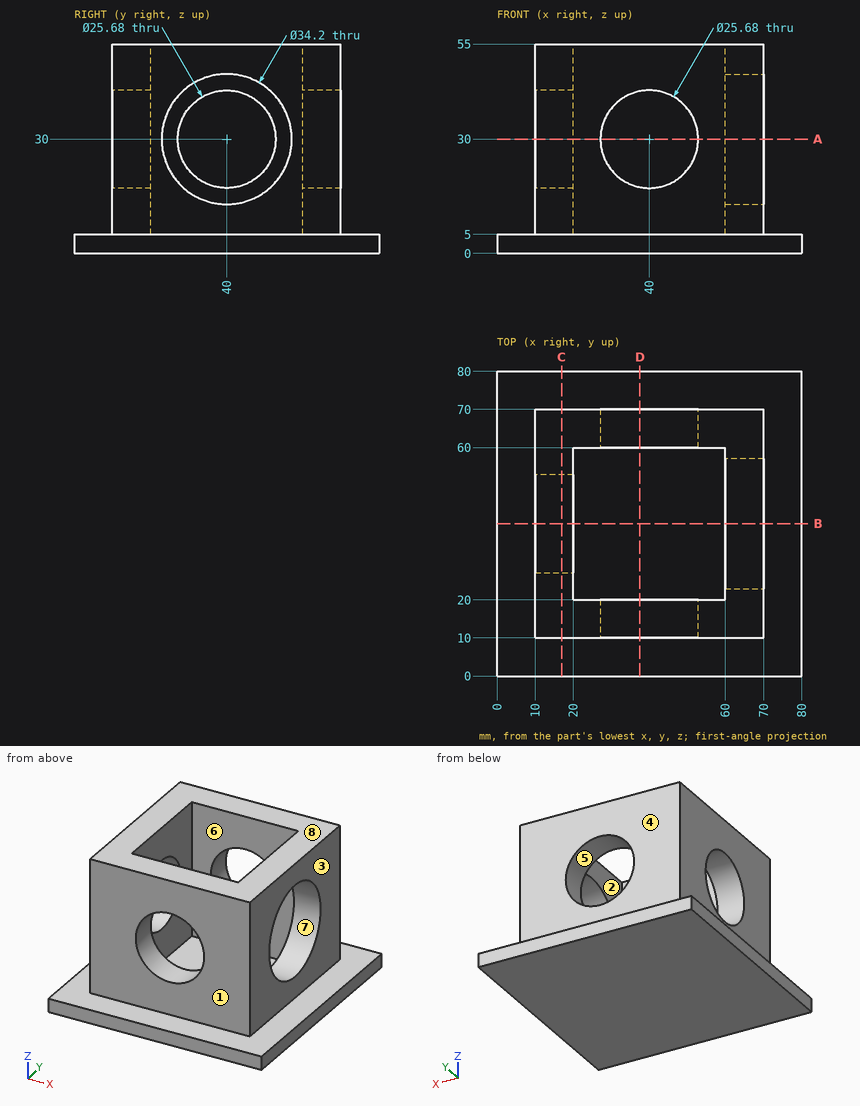
Design review of the part shown in the three views and the two pictorial views. Dimensions are in mm from the part's minimum x, y and z. A direction names the side the tool comes from. Coordinates: 2 decimals unless noted, no trailing zeros. Order: outer loops, then holes, each group sorted by start corner. A loop starts at its lowest first (then second) coordinate and runs counter-clockwise, first axis right, second up. Notation, with made-up numbers: (31.5, -11) -> (67.5, -11) arc R28 ccw to (67.5, 16) -> close; hole circle Ø5 at (57, -8.5). An arc over 180 degrees is marked (long way). Use one line per item in the form item = value. Start each with the question number.
(1) Add section D-D on x = 37.5. State the section outline as (y, z) points.
(2) The part is to be moulded in two halves that separate along Z. For the marked faces 5, 6, 7 and 8, say which applies: +Z half, -Z half, draft (parallel to the pull), parting line (faces both ways), or undercut.
(3) Add section C-C on x = 17. State the section outline as (y, z) points.
(4) For probe 1 along Y at (x, z) = (26, 40.5); probe 2 along Z at (x, y) = (63.75, 40); probe 3 along X at (y, z) = (40, 15), list the stretches that pass through material, from the lowest coordinate up.
(5) Add section B-B on y = 40. State the section outline as (x, z) points, plus the area to 3 significant figures.
(6) Insertion check: pin 1 (10 mm diameter, centred on x = 61, z = 31, fed in from -Y); pin 2 (1.5 mm diameter, centred on x = 67, y = 59.5, fed in from -Z); pin 3 (10 mm diameter, centred on y = 41, z = 48.5, fed in from +X); pin 4 (25 mm diameter, centred on x = 54.5, z = 22.5, fed in from +Y). Each pin has a flat end and moves straight along its axis. Give the tip position at first contact, or say it passes through.
(7) For the marked faces 1, 2, 3 and 4, list the 3-axis set-ups (+Z, -Z, +X, -X, +Y, -Y) from which the entire face can be reached by the end or side of a thin tool; tool diameter is ignored.
(8) Add section A-A on z = 30. State the section outline as (x, y) points, plus the area to 3 significant figures.
Answer block:
q1.outline = (0, 0) -> (80, 0) -> (80, 5) -> (70, 5) -> (70, 17.41) -> (60, 17.41) -> (60, 5) -> (20, 5) -> (20, 17.41) -> (10, 17.41) -> (10, 5) -> (0, 5) -> close; (10, 42.59) -> (20, 42.59) -> (20, 55) -> (10, 55) -> close; (60, 42.59) -> (70, 42.59) -> (70, 55) -> (60, 55) -> close
q2.face_5 = undercut
q2.face_6 = draft
q2.face_7 = undercut
q2.face_8 = +Z half
q3.outline = (0, 0) -> (80, 0) -> (80, 5) -> (70, 5) -> (70, 55) -> (10, 55) -> (10, 5) -> (0, 5) -> close; hole circle Ø25.68 at (40, 30)
q4.probe_1 = 10 to 20, 60 to 70
q4.probe_2 = 0 to 12.9, 47.1 to 55
q4.probe_3 = 10 to 20
q5.outline = (0, 0) -> (80, 0) -> (80, 5) -> (70, 5) -> (70, 12.9) -> (60, 12.9) -> (60, 5) -> (20, 5) -> (20, 17.16) -> (10, 17.16) -> (10, 5) -> (0, 5) -> close; (10, 42.84) -> (20, 42.84) -> (20, 55) -> (10, 55) -> close; (60, 47.1) -> (70, 47.1) -> (70, 55) -> (60, 55) -> close
q5.area = 801 mm²
q6.pin_1 = 10
q6.pin_2 = 0
q6.pin_3 = 70
q6.pin_4 = 70
q7.face_1 = +Z, +X, -X, -Y
q7.face_2 = +Z
q7.face_3 = +Z, +X, +Y, -Y
q7.face_4 = +Z, +X, -X, +Y
q8.outline = (10, 10) -> (27.16, 10) -> (27.16, 20) -> (20, 20) -> (20, 27.16) -> (10, 27.16) -> close; (10, 52.84) -> (20, 52.84) -> (20, 60) -> (27.16, 60) -> (27.16, 70) -> (10, 70) -> close; (52.84, 10) -> (70, 10) -> (70, 22.9) -> (60, 22.9) -> (60, 20) -> (52.84, 20) -> close; (52.84, 60) -> (60, 60) -> (60, 57.1) -> (70, 57.1) -> (70, 70) -> (52.84, 70) -> close
q8.area = 888 mm²
